```python
from build123d import *

# Parameters (mm, degrees)
SKETCH2_W           = 60
SKETCH2_H           = 24
SKETCH2_R           = 7.5
BOSS_EXTRUDE1_DEPTH = 47
SKETCH2_2_W         = 60
SKETCH2_2_H         = 24
SKETCH2_2_R         = 7.5
BOSS_EXTRUDE2_DEPTH = 25.5
SKETCH8_R           = 2
CUT_EXTRUDE1_DEPTH  = 61.704200843


with BuildPart() as part:
    # Sketch2 → Boss-Extrude1 (new body)
    with BuildSketch(Plane(origin=(0, 0, 0), x_dir=(1, 0, 0), z_dir=(0, 1, 0))):
        Rectangle(SKETCH2_W, SKETCH2_H)
        with Locations(Location((0, 0, 0), (0, 0, 270))):
            Circle(SKETCH2_R, mode=Mode.SUBTRACT)
    extrude(amount=BOSS_EXTRUDE1_DEPTH)

    # Sketch2_2 → Boss-Extrude2 (add)
    with BuildSketch(Plane(origin=(0, 0, 0), x_dir=(1, 0, 0), z_dir=(0, 1, 0))):
        Rectangle(SKETCH2_2_W, SKETCH2_2_H)
        with Locations(Location((0, 0, 0), (0, 0, 270))):
            Circle(SKETCH2_2_R, mode=Mode.SUBTRACT)
    extrude(amount=BOSS_EXTRUDE2_DEPTH)

    # Sketch8 → Cut-Extrude1 (cut, through all)
    with BuildSketch(Plane.XY.offset(12)):
        with Locations((-21, 9)):
            Circle(SKETCH8_R)
        with Locations((-21, 38)):
            Circle(SKETCH8_R)
        with Locations((21, 38)):
            Circle(SKETCH8_R)
        with Locations((21, 9)):
            Circle(SKETCH8_R)
    extrude(amount=-CUT_EXTRUDE1_DEPTH, mode=Mode.SUBTRACT)


solid = part.part
```
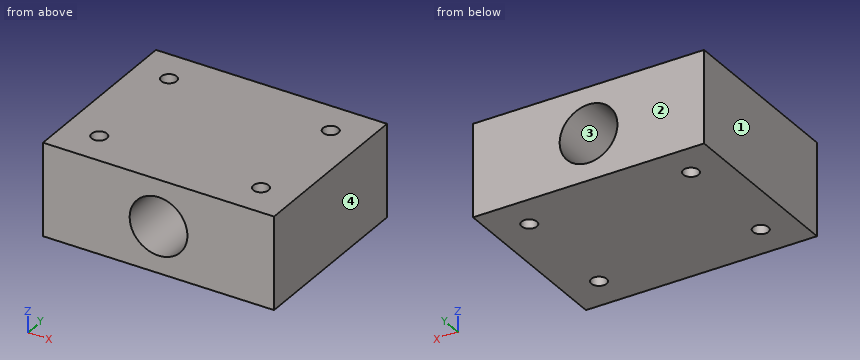
Geometry: final body of the model. Coordinates: model frame, mm. Face numbers are marked on the shaded views. Round coordinates to 2 decimals unless told otherwise and drop trailing zeros. Loops run counter-clockwise (first coordinate to the right, second up) from the corner with the lowest first, then second, coordinate; pieces in that order, holes last. Notation, with made-up numbers: (-8.5, 14.25) -> (29.5, 14.25) arc R14 cw to (29.5, 24.25) -> close; hole circle Ø1 at (-15, -19). An arc over 180 degrees is marked (long way). Write each question's results on one line, items separated by ' | '.
Item 1: Pull-direction query (X, two-part tool) for the marked faces 1, 2, 3 and 4; classes: pulls with the +X half, pulls with the -X half, needs draft (parallel to the pull), parting line crosses it, or undercut.
Answers below:
face 1: pulls with the -X half | face 2: needs draft | face 3: undercut | face 4: pulls with the +X half
Item 2: Cut plane B-B on x = -21. Return the cut outline in (y, z).
Answers below:
outline: (0, -12) -> (7, -12) -> (7, 12) -> (0, 12) -> close; (11, -12) -> (36, -12) -> (36, 12) -> (11, 12) -> close; (40, -12) -> (47, -12) -> (47, 12) -> (40, 12) -> close
Item 3: Cut plane C-C on x = 0. Return the cut outline in (y, z).
Answers below:
outline: (0, -12) -> (47, -12) -> (47, -7.5) -> (0, -7.5) -> close; (0, 7.5) -> (47, 7.5) -> (47, 12) -> (0, 12) -> close
Item 4: Cut plane A-A on y = 38. Return the cut outline in (x, z), and give its area (3 significant figures).
Answers below:
outline: (-30, -12) -> (-23, -12) -> (-23, 12) -> (-30, 12) -> close; (-19, -12) -> (19, -12) -> (19, 12) -> (-19, 12) -> close; (23, -12) -> (30, -12) -> (30, 12) -> (23, 12) -> close; hole circle Ø15 at (0, 0) | area: 1,070 mm²
Item 5: Pin query (flat end, axial travel): pin 1 Ø2.5 at (x, y) = (21, 9) entering from -Z. Return the tip coordinate at first contact, or that it passes through.
Answers below:
pin 1: passes through
Item 6: Line query: probe 1 along Y at (x, z) = (21, -3.75); probe 2 along Y at (x, z) = (21.5, 8.75); probe 3 along Z at (x, y) = (2, 20). Output: solid intervals per line, ascending. Write a range as [from, to].
Answers below:
probe 1: y = [0, 7], [11, 36], [40, 47] | probe 2: y = [0, 7.06], [10.94, 36.06], [39.94, 47] | probe 3: z = [-12, -7.23], [7.23, 12]
Item 7: Cut plane D-D on z = -1.75. Return the cut outline in (x, y).
Answers below:
outline: (-30, 0) -> (-7.29, 0) -> (-7.29, 47) -> (-30, 47) -> close; (7.29, 0) -> (30, 0) -> (30, 47) -> (7.29, 47) -> close; hole circle Ø4 at (-21, 9); hole circle Ø4 at (-21, 38); hole circle Ø4 at (21, 9); hole circle Ø4 at (21, 38)
